The model under review builds one solid part; all positions refer to its coordinate system, in mm. Face numbers are marked on the shaded views. Coordinates: 2 decimals unless noted, no trailing zeros. Order: outer loops, then holes, each group sorted by start corner. A loop starts at its lowest first (then second) coordinate and runs counter-clockwise, first axis right, second up. Notation, with made-up numbers: M 31.25,-7.5 L 47.25,-7.5 A26 ccw 47.25,28.5 Z; hole C -1.75,10.25 d7. An arc over 180 degrees is marked long. Answer as CSV lines item,"result". Start each with the question number.
Q1. Consider section D-D on y = -1. Write out the cut boundary in (x, z), and give its area (3 significant figures).
Q2. Consider section B-B on y = 3.25. Write out the cut boundary in (x, z), and give its area (3 significant figures).
Q3. Consider section C-C on x = 0. Write out the cut boundary in (y, z), and give its area (3 significant figures).
Q4. For P1, Ø4, axis at x = 2.5, y = -0.5, coming from the +Z side; P2, Ø1, axis at x = -1.5, y = 2.5, coming from the +Z side, all flat-tipped, find the tip position at first contact; note any pin that passes through.
Q5. Consider section A-A on x = -4.25. Write out the cut boundary in (y, z), and give its area (3 significant figures).
Q6. Wall thickness on L1, parallel to Z at x = -1, y = -3.25; L2, parallel to X at y = 0.25, z = 0.9: over which ranges is each line inside the solid? List them lowest first. Write a range as [from, to].
Q7. The part is to be moulded in two halves that separate along X. For the marked faces 1 and 2, say which applies: +X half, -X half, draft (parallel to the pull), parting line (faces both ways), or undercut.
from build123d import *

# Parameters (mm, degrees)
F0_W     = 10
F0_H     = 8
F1_DEPTH = 0.8
F2_R     = 0.4
F3_DEPTH = 0.6


with BuildPart() as f1:
    # F0 (on Top) → F1 (new body)
    with BuildSketch(Plane.XY):
        Rectangle(F0_W, F0_H)
    extrude(amount=F1_DEPTH)

    # F2 (on face) → F3 (join)
    with BuildSketch(Plane.XY.offset(0.8)):
        with Locations((-4.25, 3.25)):
            Circle(F2_R)
        with Locations((-4.25, 0)):
            Circle(F2_R)
        with Locations((-4.25, -3.25)):
            Circle(F2_R)
        with Locations((0, 3.25)):
            Circle(F2_R)
        with Locations((4.25, 3.25)):
            Circle(F2_R)
        with Locations((4.25, 0)):
            Circle(F2_R)
        with Locations((4.25, -3.25)):
            Circle(F2_R)
        with Locations((0, -3.25)):
            Circle(F2_R)
    extrude(amount=F3_DEPTH)


solid = f1.part
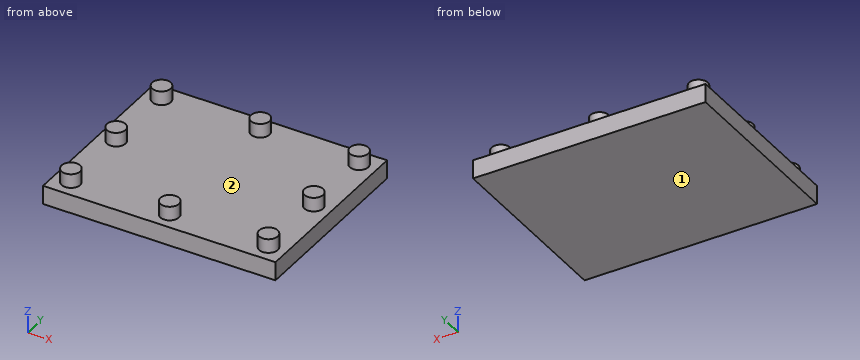
Evaluation:
1,outline,"M -5,0 L 5,0 L 5,0.8 L -5,0.8 Z"
1,area,"8.00 mm²"
2,outline,"M -5,0 L 5,0 L 5,0.8 L 4.65,0.8 L 4.65,1.4 L 3.85,1.4 L 3.85,0.8 L 0.4,0.8 L 0.4,1.4 L -0.4,1.4 L -0.4,0.8 L -3.85,0.8 L -3.85,1.4 L -4.65,1.4 L -4.65,0.8 L -5,0.8 Z"
2,area,"9.44 mm²"
3,outline,"M -4,0 L 4,0 L 4,0.8 L 3.65,0.8 L 3.65,1.4 L 2.85,1.4 L 2.85,0.8 L -2.85,0.8 L -2.85,1.4 L -3.65,1.4 L -3.65,0.8 L -4,0.8 Z"
3,area,"7.36 mm²"
4,P1,"stops at z = 1.4"
4,P2,"stops at z = 0.8"
5,outline,"M -4,0 L 4,0 L 4,0.8 L 3.65,0.8 L 3.65,1.4 L 2.85,1.4 L 2.85,0.8 L 0.4,0.8 L 0.4,1.4 L -0.4,1.4 L -0.4,0.8 L -2.85,0.8 L -2.85,1.4 L -3.65,1.4 L -3.65,0.8 L -4,0.8 Z"
5,area,"7.84 mm²"
6,L1,"z = [0, 0.8]"
6,L2,"x = [-4.56, -3.94], [3.94, 4.56]"
7,face 1,"draft"
7,face 2,"undercut"
